```python
from build123d import *

# Parameters (mm, degrees)
SKETCH1_R            = 15
BOSS_EXTRUDE1_DEPTH  = 27
SKETCH2_R            = 14
BOSS_EXTRUDE2_DEPTH  = 5
SKETCH3_R            = 5
BOSS_EXTRUDE3_DEPTH  = 3
SKETCH4_R            = 1.25
BOSS_EXTRUDE4_DEPTH  = 7
BOSS_EXTRUDE5_START  = 6
SKETCH5_R            = 14
BOSS_EXTRUDE5_DEPTH  = 6
BOSS_EXTRUDE6_START  = 3
SKETCH6_R            = 5
BOSS_EXTRUDE6_DEPTH  = 3
SKETCH7_W            = 28
SKETCH7_H            = 28
BOSS_EXTRUDE7_DEPTH  = 2.5
BOSS_EXTRUDE8_START  = 4
SKETCH8_R            = 1.25
BOSS_EXTRUDE8_DEPTH  = 4
BOSS_EXTRUDE9_START  = 1
SKETCH9_R            = 5
BOSS_EXTRUDE9_DEPTH  = 1
SKETCH10_R           = 11
BOSS_EXTRUDE10_DEPTH = 0.5
BOSS_EXTRUDE11_START = 1
SKETCH11_R           = 5
BOSS_EXTRUDE11_DEPTH = 1
BOSS_EXTRUDE12_START = 3
SKETCH12_R           = 1.25
BOSS_EXTRUDE12_DEPTH = 3


with BuildPart() as part:
    # Sketch1 → Boss-Extrude1 (new body)
    with BuildSketch(Plane(origin=(0, 0, 0), x_dir=(1, 0, 0), z_dir=(0, 1, 0))):
        with Locations(Location((0, 0, 0), (0, 0, 270))):
            Circle(SKETCH1_R)
    extrude(amount=BOSS_EXTRUDE1_DEPTH)

    # Sketch2 → Boss-Extrude2 (add)
    with BuildSketch(Plane(origin=(0, 27, 0), x_dir=(1, 0, 0), z_dir=(0, 1, 0))):
        with Locations(Location((0, 0, 0), (0, 0, 270))):
            Circle(SKETCH2_R)
    extrude(amount=BOSS_EXTRUDE2_DEPTH)

    # Sketch3 → Boss-Extrude3 (add)
    with BuildSketch(Plane(origin=(0, 32, 0), x_dir=(1, 0, 0), z_dir=(0, 1, 0))):
        with Locations(Location((0, 0, 0), (0, 0, 270))):
            Circle(SKETCH3_R)
    extrude(amount=BOSS_EXTRUDE3_DEPTH)

    # Sketch4 → Boss-Extrude4 (add)
    with BuildSketch(Plane(origin=(0, 35, 0), x_dir=(1, 0, 0), z_dir=(0, 1, 0))):
        with Locations(Location((0, 0, 0), (0, 0, 270))):
            Circle(SKETCH4_R)
    extrude(amount=BOSS_EXTRUDE4_DEPTH)

    # Sketch5 → Boss-Extrude5 (add)
    with BuildSketch(Plane.XZ.offset(BOSS_EXTRUDE5_START)):
        with Locations(Location((0, 0, 0), (0, 0, 90))):
            Circle(SKETCH5_R)
    extrude(amount=-BOSS_EXTRUDE5_DEPTH)

    # Sketch6 → Boss-Extrude6 (add)
    with BuildSketch(Plane.XZ.offset(6).offset(BOSS_EXTRUDE6_START)):
        with Locations(Location((0, 0, 0), (0, 0, 90))):
            Circle(SKETCH6_R)
    extrude(amount=-BOSS_EXTRUDE6_DEPTH)

    # Sketch7 → Boss-Extrude7 (add)
    with BuildSketch(Plane.XZ.offset(6)):
        with Locations((-14, 0)):
            Rectangle(SKETCH7_W, SKETCH7_H)
    extrude(amount=BOSS_EXTRUDE7_DEPTH)

    # Sketch8 → Boss-Extrude8 (add)
    with BuildSketch(Plane.XZ.offset(9).offset(BOSS_EXTRUDE8_START)):
        with Locations(Location((0, 0, 0), (0, 0, 90))):
            Circle(SKETCH8_R)
    extrude(amount=-BOSS_EXTRUDE8_DEPTH)

    # Sketch9 → Boss-Extrude9 (add)
    with BuildSketch(Plane.XZ.offset(13).offset(BOSS_EXTRUDE9_START)):
        with Locations(Location((0, 0, 0), (0, 0, 270))):
            Circle(SKETCH9_R)
    extrude(amount=-BOSS_EXTRUDE9_DEPTH)

    # Sketch10 → Boss-Extrude10 (add)
    with BuildSketch(Plane.XZ.offset(14)):
        with Locations(Location((0, 0, 0), (0, 0, 270))):
            Circle(SKETCH10_R)
    extrude(amount=BOSS_EXTRUDE10_DEPTH)

    # Sketch11 → Boss-Extrude11 (add)
    with BuildSketch(Plane.XZ.offset(14.5).offset(BOSS_EXTRUDE11_START)):
        with Locations(Location((0, 0, 0), (0, 0, 270))):
            Circle(SKETCH11_R)
    extrude(amount=-BOSS_EXTRUDE11_DEPTH)

    # Sketch12 → Boss-Extrude12 (add)
    with BuildSketch(Plane.XZ.offset(15.5).offset(BOSS_EXTRUDE12_START)):
        with Locations(Location((0, 0, 0), (0, 0, 90))):
            Circle(SKETCH12_R)
    extrude(amount=-BOSS_EXTRUDE12_DEPTH)


solid = part.part
```
For this review, take the finished solid that the model builds, in its own axes (mm). A direction names the side the tool comes from. Coordinates: 2 decimals unless noted, no trailing zeros. Write each loop counter-clockwise with the first axis right and the second up, starting at its lowest first coordinate (ties: lowest second). Pieces come first, ordered by that corner, then holes. Notation, with made-up numbers: (79.5, 10) - (90.5, 10) arc R15 ccw to (90.5, 14) - close; hole circle Ø11 at (67, -9.5). An arc over 180 degrees is marked (long way). Answer in a Markdown table with one row per item. Add a question column.
Q1. We need section B-B, the plane z = 8.75. State the section outline as (x, y) points.
Q2. Draft analysis for pull direction Y (two halves, no side actions). For faces 6 (the flat face through (-14, -8.5, 0)), 7 (the cylindrical face through (1.22, -17.02, -0.27)), 8 (the flat face through (1, -9, 1)), 9 (the flat face through (-1, -15.5, -1)), state which applies: +Y half, -Y half, draft (parallel to the pull), parting line (faces both ways), or undercut.
Q3. Tool access review of faces 1 (the cylindrical face through (4.88, -7.85, -1.08)), 2 (the flat face through (-14, -7, -14)), 3 (the cylindrical face through (-4.88, 33.48, -1.08)), 4 (the flat face through (0, -7, -10)), 5 (the flat face through (7, -6, 0)): name each direction out of +Z, -Z, +X, -X, +Y, -Y from which nothing blocks a thin tool from reaching the whole face with its end or side.
Q4. For probe 1 along Y at (x, z) = (3, 5); probe 2 along Y at (x, z) = (-4, -12.75); probe 3 along Y at (x, z) = (-12.5, -12.75), list the stretches that pass through material, from the lowest coordinate up.
Q5. We need section C-C, the plane y = 38.5. State the section outline as (x, z) points.
Q6. For P1, Ø5, axis at x = 10, z = 5, coming from the -Y side; P2, Ø12, axis at x = -20, y = -8, coming from the +Z side; P3, Ø9, axis at x = -7, z = -2, coming from the +Y side, all flat-tipped, find the tip position at first contact; note any pin that passes through.
Q7. We need section A-A, the plane x = 8. State the section outline as (y, z) points.
Answer list:
| question | item | result |
|---|---|---|
| 1 | outline | (-28, -8.5) - (0, -8.5) - (0, -6) - (10.93, -6) - (10.93, 0) - (12.18, 0) - (12.18, 27) - (10.93, 27) - (10.93, 32) - (-10.93, 32) - (-10.93, 27) - (-12.18, 27) - (-12.18, 0) - (-10.93, 0) - (-10.93, -6) - (-28, -6) - close; (-6.67, -14.5) - (6.67, -14.5) - (6.67, -14) - (-6.67, -14) - close |
| 2 | face 6 | undercut |
| 2 | face 7 | draft |
| 2 | face 8 | undercut |
| 2 | face 9 | -Y half |
| 3 | face 1 | none |
| 3 | face 2 | -Z, +X, -X, -Y |
| 3 | face 3 | +Y |
| 3 | face 4 | -Z, +X |
| 3 | face 5 | +X |
| 4 | probe 1 | y = -14.5 to -14, -6 to 32 |
| 4 | probe 2 | y = -8.5 to 32 |
| 4 | probe 3 | y = -8.5 to -6 |
| 5 | outline | circle Ø2.5 at (0, 0) |
| 6 | P1 | stops at y = -14.5 |
| 6 | P2 | stops at z = 14 |
| 6 | P3 | stops at y = 35 |
| 7 | outline | (-14.5, -7.55) - (-14, -7.55) - (-14, 7.55) - (-14.5, 7.55) - close; (-6, -11.49) - (0, -11.49) - (0, -12.69) - (27, -12.69) - (27, -11.49) - (32, -11.49) - (32, 11.49) - (27, 11.49) - (27, 12.69) - (0, 12.69) - (0, 11.49) - (-6, 11.49) - close |
